from build123d import *

# Parameters (mm, degrees)
F0_R     = 1.5
F1_DEPTH = 26
F2_R     = 1.4
F3_DEPTH = 0.5
F4_R     = 1.4
F5_DEPTH = 0.5
F6_R     = 1.5
F7_DEPTH = 2.5
F8_R     = 1.5
F9_DEPTH = 2.5


with BuildPart() as f1:
    # F0 (on Right) → F1 (new body)
    with BuildSketch(Plane.YZ):
        Circle(F0_R)
    extrude(amount=F1_DEPTH)

    # F2 (on face) → F3 (join)
    with BuildSketch(Plane.YZ.offset(26)):
        Circle(F2_R)
    extrude(amount=F3_DEPTH)

    # F4 (on face) → F5 (join)
    with BuildSketch(Plane(origin=(0, 0, 0), x_dir=(0, -1, 0), z_dir=(-1, 0, 0))):
        Circle(F4_R)
    extrude(amount=F5_DEPTH)

    # F6 (on face) → F7 (join)
    with BuildSketch(Plane(origin=(-0.5, 0, 0), x_dir=(0, -1, 0), z_dir=(-1, 0, 0))):
        Circle(F6_R)
    extrude(amount=F7_DEPTH)

    # F8 (on face) → F9 (join)
    with BuildSketch(Plane.YZ.offset(26.5)):
        Circle(F8_R)
    extrude(amount=F9_DEPTH)


solid = f1.part
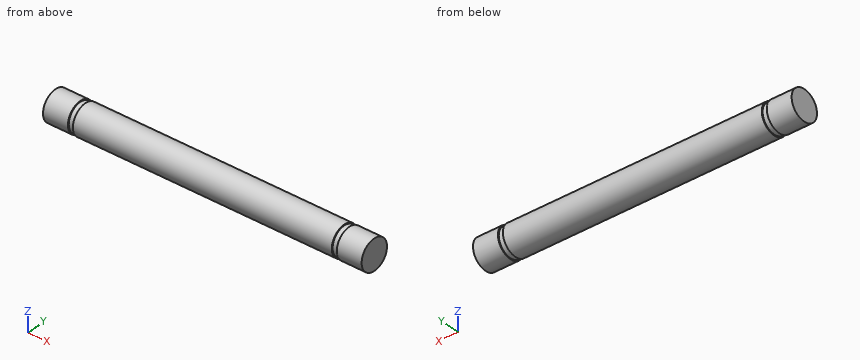
Geometry check sheet. Reference: the model listing, model coordinates, mm. Give positions to 0.01 mm unless a question says otherwise; leave off trailing zeros. Order: outer loops, then holes, each group sorted by start corner. A loop starts at its lowest first (then second) coordinate and runs counter-clockwise, first axis right, second up. Notation, with made-up numbers: M 58,-21 L 79,-21 A7 ccw 79,-8 Z; hole C 72,63 d11. An arc over 180 degrees is marked long. Use a Markdown table: item, result.
Item 1: Material ranges on line 1 along X through (y, z) = (0.7, 1.25); line 2 along Y through (x, z) = (13, -0.1); line 3 along Y through (x, z) = (16.5, 0.55), recorded low to high.
Answers follow:
| item | result |
|---|---|
| line 1 | x = -3 to -0.5, 0 to 26, 26.5 to 29 |
| line 2 | y = -1.5 to 1.5 |
| line 3 | y = -1.4 to 1.4 |
Item 2: Depth check by flat-ended pin: P1, Ø1.5, axis at x = 2, z = 0.5, coming from the +Y side. Enter the tip coordinate at first touch or a pass-through.
Answers follow:
| item | result |
|---|---|
| P1 | stops at y = 1.5 |
Item 3: Section check A-A (z = 0.4). Record the cut outline in (x, y), and give its area (3 significant figures).
Answers follow:
| item | result |
|---|---|
| outline | M -3,-1.45 L -0.5,-1.45 L -0.5,-1.34 L 0,-1.34 L 0,-1.45 L 26,-1.45 L 26,-1.34 L 26.5,-1.34 L 26.5,-1.45 L 29,-1.45 L 29,1.45 L 26.5,1.45 L 26.5,1.34 L 26,1.34 L 26,1.45 L 0,1.45 L 0,1.34 L -0.5,1.34 L -0.5,1.45 L -3,1.45 Z |
| area | 92.3 mm2 |
Item 4: Section check B-B (x = 1.5). Record the cut outline in (y, z).
Answers follow:
| item | result |
|---|---|
| outline | C 0,0 d3 |
Item 5: Section check C-C (y = -0.45). Record the cut outline in (x, z), and give its area (3 significant figures).
Answers follow:
| item | result |
|---|---|
| outline | M -3,-1.43 L -0.5,-1.43 L -0.5,-1.33 L 0,-1.33 L 0,-1.43 L 26,-1.43 L 26,-1.33 L 26.5,-1.33 L 26.5,-1.43 L 29,-1.43 L 29,1.43 L 26.5,1.43 L 26.5,1.33 L 26,1.33 L 26,1.43 L 0,1.43 L 0,1.33 L -0.5,1.33 L -0.5,1.43 L -3,1.43 Z |
| area | 91.4 mm2 |
